Here's how the part is built. I have some questions about the finished solid (model axes, mm). Face numbers are marked on the shaded views. Round coordinates to 2 decimals unless told otherwise and drop trailing zeros. Write each loop counter-clockwise with the first axis right and the second up, starting at its lowest first coordinate (ties: lowest second). Pieces come first, ordered by that corner, then holes. Notation, with made-up numbers: M -2,87.5 L 42,87.5 A29 cw 42,121.5 Z; hole C -26.75,62.25 d9. An arc over 180 degrees is marked long. Use one line per item in the form item = value. Start each with the question number.
Q1. I'm going to push flat-ended pins straight in: pin 1 Ø3 at (x, y) = (2.5, 11.5) entering from -Z; pin 2 Ø1 at (x, z) = (9.5, -7.5) entering from -Y; pin 3 Ø2 at (x, z) = (9.5, -2) entering from +Y. Where does each tip first touch, or does it pass through?
Q2. I want a section at A-A on y = 0. List the corners of the cut face in (x, z) for me.
Q3. I need wall thicknesses on line 1 along Z through (x, y) = (5.5, 0); line 2 along Z through (x, y) = (6.25, -45); line 3 along Y through (x, z) = (3.5, 35). Which ranges of each line are inside material? Lowest first, please. Write a range as from..to.
Q4. I want a section at B-B on x = 8. State how many separate pieces and enclosed holes the cut face has, and give its area (3 significant figures).
Q5. I want a section at D-D on z = 35.5. List the corners of the cut face in (x, y) for me (3 decimals), and give its area (3 significant figures).
Q6. We'd pull the mould along Z, two halves only. Please class the marked faces 1, 2 and 3: +Z half, -Z half, draft (parallel to the pull), parting line (faces both ways), or undercut.
Q7. I want a section at C-C on y = 22.5. List the corners of the cut face in (x, z) for me, and give its area (3 significant figures).
```python
from build123d import *

# Parameters (mm, degrees)
SKETCH1_R           = 49
SKETCH1_R_2         = 41
BOSS_EXTRUDE1_DEPTH = 12
CIRPATTERN1_COUNT   = 6
CUT_EXTRUDE1_START  = -12
CUT_EXTRUDE1_DEPTH  = 12
FILLET1_R           = 4


with BuildPart() as part:
    # Sketch1 → Boss-Extrude1 (new body)
    with BuildSketch(Plane(origin=(0, 0, 0), x_dir=(0, 0, -1), z_dir=(1, 0, 0))):
        Circle(SKETCH1_R)
        Circle(SKETCH1_R_2, mode=Mode.SUBTRACT)
    extrude(amount=BOSS_EXTRUDE1_DEPTH)

    # Sketch3 → Ø4.0mm Dowel Hole1 (revolve, cut)
    with BuildSketch(Plane(origin=(12, 45, 0), x_dir=(0, 0, -1), z_dir=(0, 1, 0))):
        Polygon((0, 0), (0, 51.201721238), (2, 50), (2, 0), align=None)
    f_4_0mm_dowel_hole1 = revolve(axis=Axis((18.35, 45, 0), (-1, 0, 0)), mode=Mode.SUBTRACT)

    # CirPattern1: Ø4.0mm Dowel Hole1 ×6 about axis
    cirpattern1_axis = Axis((0, 0, 0), (1, 0, 0))
    for i in range(1, CIRPATTERN1_COUNT):
        add(f_4_0mm_dowel_hole1.rotate(cirpattern1_axis, i * 360 / CIRPATTERN1_COUNT), mode=Mode.SUBTRACT)

    # Sketch4 → Cut-Extrude1 (cut)
    with BuildSketch(Plane(origin=(12, 0, 0), x_dir=(0, 0, -1), z_dir=(1, 0, 0)).offset(CUT_EXTRUDE1_START)):
        with BuildLine():
            Line((-36.670833097, 32.5), (0, 0))
            Line((0, 0), (36.670833097, 32.5))
            ThreePointArc((36.670833097, 32.5), (0, 49), (-36.670833097, 32.5))
        make_face()
    extrude(amount=CUT_EXTRUDE1_DEPTH, mode=Mode.SUBTRACT)

    # Fillet1
    fillet1_edges = [part.edges().sort_by_distance(p)[0] for p in [
        (6, 32.5, -36.670833097),
        (6, 27.193877551, -30.683758305),
        (6, 27.193877551, 30.683758305),
        (6, 32.5, 36.670833097),
    ]]
    fillet(fillet1_edges, radius=FILLET1_R - 0.0001)  # a hair under: the kernel refuses the full size


solid = part.part
```
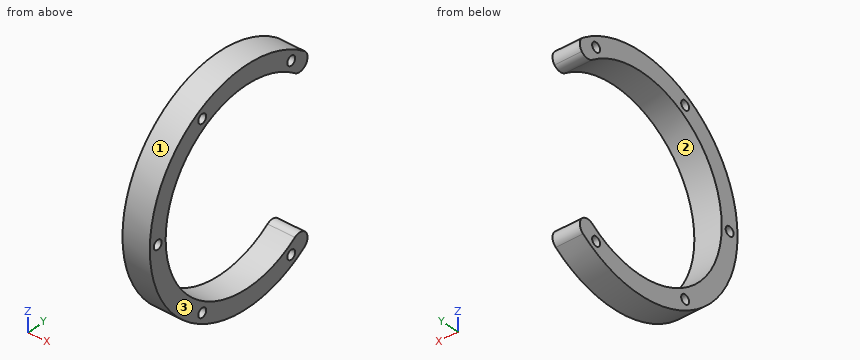
Reported:
q1.pin_1 = -47.97
q1.pin_2 = -48.5
q1.pin_3 = -40.89
q2.outline = M 0,-49 L 12,-49 L 12,-41 L 0,-41 Z; M 0,41 L 12,41 L 12,49 L 0,49 Z
q3.line_1 = -49..-41, 41..49
q3.line_2 = -19.39..-2, 2..19.39
q3.line_3 = -34.29..-21.35, 21.35..30.55
q4.separate_pieces = 1
q4.enclosed_holes = 5
q4.area = 1,580 mm^2
q5.outline = M 0,-33.775 L 12,-33.775 L 12,-20.512 L 0,-20.512 Z; M 0,20.512 L 12,20.512 L 12,30.674 L 0,30.674 Z
q5.area = 281 mm^2
q6.face_1 = parting line
q6.face_2 = undercut
q6.face_3 = draft
q7.outline = M 0,-43.53 L 12,-43.53 L 12,-40.97 L 0,-40.97 Z; M 0,-36.97 L 12,-36.97 L 12,-34.27 L 0,-34.27 Z; M 0,34.27 L 12,34.27 L 12,36.97 L 0,36.97 Z; M 0,40.97 L 12,40.97 L 12,43.53 L 0,43.53 Z
q7.area = 126 mm^2
